from build123d import *

# Parameters (mm, degrees)
SKETCH1_W           = 40
SKETCH1_H           = 47
BOSS_EXTRUDE1_DEPTH = 15
SKETCH2_W           = 28
SKETCH2_H           = 17
SKETCH2_W_2         = 24
SKETCH2_H_2         = 13
BOSS_EXTRUDE2_DEPTH = 12
SKETCH4_W           = 7.067405003
SKETCH4_H           = 7.5
CUT_EXTRUDE1_DEPTH  = 2


with BuildPart() as part:
    # Sketch1 → Boss-Extrude1 (new body)
    with BuildSketch(Plane(origin=(0, 0, 0), x_dir=(0, 0, -1), z_dir=(1, 0, 0))):
        Rectangle(SKETCH1_W, SKETCH1_H)
    extrude(amount=BOSS_EXTRUDE1_DEPTH)

    # Sketch2 → Boss-Extrude2 (add)
    with BuildSketch(Plane(origin=(15, 0, 0), x_dir=(0, 0, -1), z_dir=(1, 0, 0))):
        with Locations((-5.5, 15)):
            Rectangle(SKETCH2_W, SKETCH2_H)
        with Locations((-5.5, 15)):
            Rectangle(SKETCH2_W_2, SKETCH2_H_2, mode=Mode.SUBTRACT)
    extrude(amount=BOSS_EXTRUDE2_DEPTH)

    # Sketch4 → Cut-Extrude1 (cut)
    with BuildSketch(Plane(origin=(0, 23.5, 0), x_dir=(1, 0, 0), z_dir=(0, 1, 0))):
        with Locations((3.533702502, -1.707739217)):
            Rectangle(SKETCH4_W, SKETCH4_H)
    extrude(amount=-CUT_EXTRUDE1_DEPTH, mode=Mode.SUBTRACT)


solid = part.part
Could you check a few things on this model? Use its own coordinates, in mm. A direction names the side the tool comes from. Give positions to 0.01 mm unless a question says otherwise; leave off trailing zeros. Loops run counter-clockwise (first coordinate to the right, second up) from the corner with the lowest first, then second, coordinate; pieces in that order, holes last. Notation, with made-up numbers: (81, 70.5) -> (92, 70.5) arc R22 ccw to (92, 79.5) -> close; hole circle Ø4 at (2, 56). An arc over 180 degrees is marked (long way). Return JSON: item names as keys, results as strings.
Item 1: If we section it at D-D on z = -11.5: List the corners of the cut face in (x, y) for me, plus the area to 3 significant figures.
Geometry results:
{"outline": "(0, -23.5) -> (15, -23.5) -> (15, 23.5) -> (0, 23.5) -> close", "area": "705 mm²"}
Item 2: We'd pull the mould along Z, two halves only. Please class faces 6 (the flat face through (0, 0, 0)), 7 (the flat face through (21, 8.5, 6)), 8 (the flat face through (21, 15, -8.5)): +Z half, -Z half, draft (parallel to the pull), parting line (faces both ways), or undercut.
Geometry results:
{"face 6": "draft", "face 7": "undercut", "face 8": "-Z half"}
Item 3: Which directions (+Z, -Z, +X, -X, +Y, -Y) give clear straight access to the entire face, cutting with the end or side of a thin tool? Please do faces 1 (the flat face through (21, 6.5, 6)), 2 (the flat face through (15, 15, 6)), 3 (the flat face through (3, 23, -2.042)), 4 (the flat face through (13, 23.5, 5)), 5 (the flat face through (21, 15, 19.5)).
Geometry results:
{"face 1": "+Z, -Z, +X, -Y", "face 2": "+X", "face 3": "-X, +Y", "face 4": "+Z, -Z, +X, -X, +Y", "face 5": "+Z, +X, +Y, -Y"}
Item 4: I need wall thicknesses on L1, parallel to Y at x = 22.75, z = 17; L2, parallel to X at y = -10, z = -11; L3, parallel to Y at x = 3, z = 0.5. Which ranges of each line are inside material? Lowest first, please. Write a range as from..to.
Geometry results:
{"L1": "y = 6.5..8.5, 21.5..23.5", "L2": "x = 0..15", "L3": "y = -23.5..21.5"}
Item 5: If we section it at C-C on z = 11: List the corners of the cut face in (x, y) for me, plus the area to 3 significant figures.
Geometry results:
{"outline": "(0, -23.5) -> (15, -23.5) -> (15, 6.5) -> (27, 6.5) -> (27, 8.5) -> (15, 8.5) -> (15, 21.5) -> (27, 21.5) -> (27, 23.5) -> (0, 23.5) -> close", "area": "753 mm²"}
Item 6: If we section it at A-A on x = 19.75: List the corners of the cut face in (y, z) for me.
Geometry results:
{"outline": "(6.5, -8.5) -> (23.5, -8.5) -> (23.5, 19.5) -> (6.5, 19.5) -> close; hole (8.5, -6.5) -> (21.5, -6.5) -> (21.5, 17.5) -> (8.5, 17.5) -> close"}
Item 7: I'm going to push flat-ended pins straight in: pin 1 (9.5 mm diameter, centred on x = 21.5, y = 15.5, fed in from -Z); pin 2 (6 mm diameter, centred on x = 21, z = 5, fed in from -Y); pin 3 (1.5 mm diameter, centred on y = -1, z = 5, fed in from +X); pin 4 (13 mm diameter, centred on x = 20.5, z = 11.5, fed in from -Y). Where does each tip first touch, or does it pass through?
Geometry results:
{"pin 1": "stops at z = -8.5", "pin 2": "stops at y = 6.5", "pin 3": "stops at x = 15", "pin 4": "stops at y = -23.5"}
Item 8: If we section it at B-B on y = 9.5: List the corners of the cut face in (x, z) for me.
Geometry results:
{"outline": "(0, -20) -> (15, -20) -> (15, -8.5) -> (27, -8.5) -> (27, -6.5) -> (15, -6.5) -> (15, 17.5) -> (27, 17.5) -> (27, 19.5) -> (15, 19.5) -> (15, 20) -> (0, 20) -> close"}
